Autodesk Inventor part; units mm, degrees
ref_plane "YZ Plane" through (0, 0, 0) normal (1, 0, 0) x (0, 1, 0)
ref_plane "XZ Plane" through (0, 0, 0) normal (0, 1, 0) x (-1, 0, 0)
ref_plane "XY Plane" through (0, 0, 0) normal (0, 0, 1) x (1, 0, 0)
sketch "Szkic1" plane through (0, 0, 0) normal (0, 0, 1) x (1, 0, 0)
  circle A0 centre (0, 0) radius 2.5
  circle A1 centre (0, 0) radius 5
  dimension "d0" = 5
  dimension "d1" = 10
extrude "Wyciągnięcie proste1" add sketch "Szkic1" along normal mid plane 5
fillet "Zaokrąglenie1" radius 0.25 2 edges at (-5, 0, 2.5) (-5, 0, -2.5)
properties part number "magnes-N35H" material "Magnez"
Here's how the part is built. I have some questions about the finished solid (model axes, mm). Round coordinates to 2 decimals unless told otherwise and drop trailing zeros. Loops run counter-clockwise (first coordinate to the right, second up) from the corner with the lowest first, then second, coordinate; pieces in that order, holes last.
1. If I drill on line 1 along Y through (x, z) = (0, 1.45); line 2 along X through (y, z) = (-2, 1.2); line 3 along X through (y, z) = (-1.75, -1.4), over which ranges is the centre line in solid material (lowest first)?
Answer list:
line 1: y = -5 to -2.5, 2.5 to 5
line 2: x = -4.58 to -1.5, 1.5 to 4.58
line 3: x = -4.68 to -1.79, 1.79 to 4.68
2. If we section it at A-A on x = 0: Write out the boundary of the cut face in (y, z), plus the area to 3 significant figures.
Answer list:
outline: (-5, -2.25) arc R0.25 ccw to (-4.75, -2.5) - (-2.5, -2.5) - (-2.5, 2.5) - (-4.75, 2.5) arc R0.25 ccw to (-5, 2.25) - close; (2.5, -2.5) - (4.75, -2.5) arc R0.25 ccw to (5, -2.25) - (5, 2.25) arc R0.25 ccw to (4.75, 2.5) - (2.5, 2.5) - close
area: 24.9 mm2
3. For P1, Ø1, axis at y = -3.5, z = 0.5, coming from the -X side; P2, Ø3, axis at x = -3.5, z = 1, coming from the -Y side; P3, Ø3, axis at y = 2, z = -0.5, coming from the +X side, each with a flat end and sliding along its axis, tell me the tip position at first contact or that it passes through.
Answer list:
P1: stops at x = -4
P2: stops at y = -4.58
P3: stops at x = 4.97
4. We'd pull the mould along Y, two halves only. Please class faces 1 (the face through (2, -2, -2.5)), 2 (the face through (-1.08, 4.88, -0.03)), 3 (the face through (-0.54, 2.44, -0.04)): +Y half, -Y half, draft (parallel to the pull), parting line (faces both ways), or undercut.
Answer list:
face 1: draft
face 2: parting line
face 3: undercut
5. If we section it at C-C on z = 1.2: Write out the boundary of the cut face in (x, y).
Answer list:
outline: circle Ø10 at (0, 0); hole circle Ø5 at (0, 0)
